from build123d import *

# Parameters (mm, degrees)
SKETCH5_W = 73.9394
SKETCH5_H = 8.0645


with BuildPart() as part:
    # Sketch1 → Revolve1 (revolve)
    with BuildSketch(Plane.XY):
        Polygon((-38.8874, 0), (-38.8874, 24.8158), (-38.1254, 25.5778), (-31.496, 25.5778), (-30.4292, 24.511), (-29.3624, 24.511), (-29.3624, 25.781), (-28.6004, 26.543), (-0.762, 26.543), (0, 25.781), (0, 0), align=None)
    revolve(axis=Axis((0, 0, 0), (-1, 0, 0)))

    # Sketch2 → Revolve2 (revolve)
    with BuildSketch(Plane.XY):
        with BuildLine():
            Line((0, 0), (0, 15.84325))
            Line((0, 15.84325), (2.794, 15.84325))
            Line((2.794, 15.84325), (2.794, 15.6337))
            ThreePointArc((2.794, 15.6337), (3.195732339, 14.663832339), (4.1656, 14.2621))
            Line((4.1656, 14.2621), (5.477064678, 14.2621))
            ThreePointArc((5.477064678, 14.2621), (6.001953274, 14.366506833), (6.446932339, 14.663832339))
            Line((6.446932339, 14.663832339), (7.6581, 15.875))
            Line((7.6581, 15.875), (24.14016, 15.875))
            Line((24.14016, 15.875), (25.4, 14.61516))
            Line((25.4, 14.61516), (25.4, 0))
            Line((25.4, 0), (0, 0))
        make_face()
    revolve(axis=Axis((25.4, 0, 0), (-1, 0, 0)))

    # Sketch3 → Cut-Revolve1 (revolve, cut)
    with BuildSketch(Plane(origin=(0, 0, 0), x_dir=(1, 0, 0), z_dir=(0, 1, 0))):
        Polygon((-18.288, 0), (-12.612335918, -3.276846186), (-11.915865896, -25.585630358), (-10.958496254, -26.543), (-10.958496254, -29.083), (-18.288, -29.083), align=None)
    revolve(axis=Axis((-18.288, 0, 29.083), (0, 0, -1)), mode=Mode.SUBTRACT)

    # Sketch4 → Revolve3 (revolve)
    with BuildSketch(Plane.XY):
        with BuildLine():
            Line((-30.94380107, 26.318757951), (-28.812753898, 24.18771078))
            Line((-28.812753898, 24.18771078), (-28.489464678, 24.511))
            Line((-28.489464678, 24.511), (-30.470664678, 26.4922))
            Line((-30.470664678, 26.4922), (-30.871959021, 26.4922))
            ThreePointArc((-30.871959021, 26.4922), (-30.965825181, 26.429480637), (-30.94380107, 26.318757951))
        make_face()
    revolve(axis=Axis((-30.470664678, 0, 0), (-1, 0, 0)))

    # Sketch5 → Cut-Revolve2 (revolve, cut)
    with BuildSketch(Plane.XY):
        with Locations((-1.9177, 4.03225)):
            Rectangle(SKETCH5_W, SKETCH5_H)
    revolve(axis=Axis((35.052, 0, 0), (-1, 0, 0)), mode=Mode.SUBTRACT)


solid = part.part
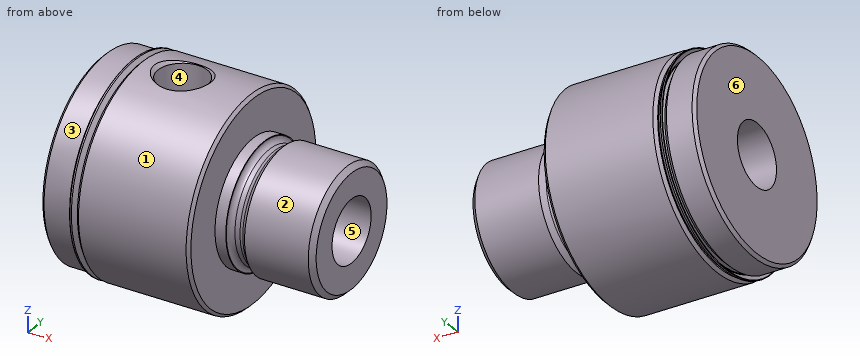
The listing builds one solid part. Answer for the finished solid, in the listing's coordinates (mm). Face numbers are marked on the shaded views. A direction names the side the tool comes from. Round coordinates to 2 decimals unless told otherwise and drop trailing zeros. Order: outer loops, then holes, each group sorted by start corner. A loop starts at its lowest first (then second) coordinate and runs counter-clockwise, first axis right, second up. Notation, with made-up numbers: (0.25, 42) - (32.25, 42) arc R26 ccw to (32.25, 66) - close; hole circle Ø11 at (51, 72). An arc over 180 degrees is marked (long way). Write item = value, one per line. Start each with the question number.
1) For a pull along Y with two mould halves and no side action, classify the marked faces 3, 4, 5 and 6 as released by +Y, released by -Y, zero draft, split by the parting line, or undercut.
2) Given pin 1 (1 mm diameter, centred on x = -20, z = 10, fed in from -Y); pin 2 (5 mm diameter, centred on x = 4, y = 11.5, fed in from -Z); pin 3 (2 mm diameter, centred on x = 4.5, z = 3, fed in from +Y), each flat-ended and moving along its own axis, determine where each tip first touches the part or whether it passes through.
3) Section B-B, the plane y = 3 is taken. Count the separate pieces of the cut face and the enclosed holes in it, plus the area to 3 significant figures.
4) Section A-A, the plane x = -33.5 is taken. Write down the section's boundary in (y, z).
5) For the marked faces 1 and 2, determine the directions among +Z, -Z, +X, -X, +Y, -Y from which every point of the face is accessible in a straight line to the end or side of a thin tool.
6) Straight lines are drawn through the part: L1, parallel to Y at x = -1, z = 0; L2, parallel to Y at x = 9, z = 0 (1 decimal). For each, find the intervals that lie inside material, in ascending order.
7) Section C-C, the plane x = -10 is taken. Write down the section's boundary in (y, z), plus the area to 3 significant figures.
Results list:
q1.face_3 = split by the parting line
q1.face_4 = undercut
q1.face_5 = undercut
q1.face_6 = zero draft
q2.pin_1 = -24.78
q2.pin_2 = -12.82
q2.pin_3 = 14.16
q3.separate_pieces = 3
q3.enclosed_holes = 0
q3.area = 1,640 mm^2
q4.outline = circle Ø51.16 at (0, 0); hole circle Ø16.13 at (0, 0)
q5.face_1 = +X, -X
q5.face_2 = +X
q6.L1 = -26.54 to -8.06, 8.06 to 26.54
q6.L2 = -15.9 to -8.1, 8.1 to 15.9
q7.outline = circle Ø53.09 at (0, 0); hole circle Ø16.13 at (0, 0)
q7.area = 2,010 mm^2
